The model under review builds one solid part; all positions refer to its coordinate system, in mm. Face numbers are marked on the shaded views. A direction names the side the tool comes from. Give positions to 0.01 mm unless a question says otherwise; leave off trailing zeros. Write each loop counter-clockwise with the first axis right and the second up, starting at its lowest first coordinate (ties: lowest second). Pieces come first, ordered by that corner, then holes. Notation, with made-up numbers: (80, 83) - (132, 83) arc R25 cw to (132, 101) - close; hole circle Ø11 at (33.25, 10.5). An arc over 180 degrees is marked (long way). Write item = value, one per line.
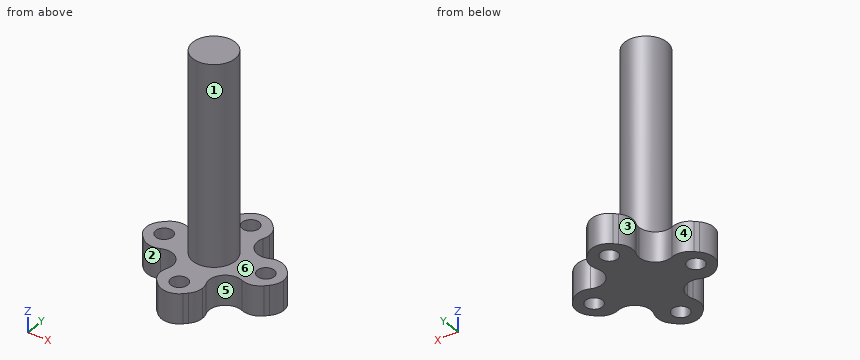
```python
from build123d import *

# Parameters (mm, degrees)
EXTRUDE_1_DEPTH = 3.5
SKETCH_3_R      = 2.5
EXTRUDE_2_DEPTH = 23.5


with BuildPart() as part:
    # 草图1 → 凸台-拉伸1 (new body)
    with BuildSketch(Plane.XY):
        with BuildLine():
            Line((-1.734039986, 7.089233915), (-1.356062107, 7.467211795))
            ThreePointArc((-1.356062107, 7.467211795), (0.128862134, 8.082287554), (1.613786374, 7.467211795))
            Line((1.613786374, 7.467211795), (1.991764254, 7.089233915))
            ThreePointArc((1.991764254, 7.089233915), (2.446987032, 6.407944883), (2.606840013, 5.604309675))
            ThreePointArc((2.606840013, 5.604309675), (2.564770676, 5.186073633), (2.440248217, 4.784594652))
            ThreePointArc((2.440248217, 4.784594652), (2.846019421, 2.699444842), (4.931169231, 2.293673637))
            ThreePointArc((4.931169231, 2.293673637), (6.152020505, 2.421597457), (7.235808495, 1.845189674))
            Line((7.235808495, 1.845189674), (7.613786374, 1.467211795))
            ThreePointArc((7.613786374, 1.467211795), (8.069009152, 0.785922762), (8.228862134, -0.017712446))
            ThreePointArc((8.228862134, -0.017712446), (8.069009152, -0.821347654), (7.613786374, -1.502636686))
            Line((7.613786374, -1.502636686), (7.235808495, -1.880614566))
            ThreePointArc((7.235808495, -1.880614566), (6.152020505, -2.457022348), (4.931169231, -2.329098529))
            ThreePointArc((4.931169231, -2.329098529), (2.846019421, -2.734869733), (2.440248217, -4.820019543))
            ThreePointArc((2.440248217, -4.820019543), (2.564770676, -5.221498525), (2.606840013, -5.639734566))
            ThreePointArc((2.606840013, -5.639734566), (2.446987032, -6.443369774), (1.991764254, -7.124658807))
            Line((1.991764254, -7.124658807), (1.613786374, -7.502636686))
            ThreePointArc((1.613786374, -7.502636686), (0.128862134, -8.117712446), (-1.356062107, -7.502636686))
            Line((-1.356062107, -7.502636686), (-1.734039986, -7.124658807))
            ThreePointArc((-1.734039986, -7.124658807), (-2.310447768, -6.040870817), (-2.182523949, -4.820019543))
            ThreePointArc((-2.182523949, -4.820019543), (-2.069860771, -4.456776655), (-2.031798038, -4.078372618))
            ThreePointArc((-2.031798038, -4.078372618), (-2.882781632, -2.494212089), (-4.673444964, -2.329098529))
            ThreePointArc((-4.673444964, -2.329098529), (-5.894296238, -2.457022348), (-6.978084227, -1.880614566))
            Line((-6.978084227, -1.880614566), (-7.356062107, -1.502636686))
            ThreePointArc((-7.356062107, -1.502636686), (-7.971137866, -0.017712446), (-7.356062107, 1.467211795))
            Line((-7.356062107, 1.467211795), (-6.978084227, 1.845189674))
            ThreePointArc((-6.978084227, 1.845189674), (-5.894296238, 2.421597457), (-4.673444964, 2.293673637))
            ThreePointArc((-4.673444964, 2.293673637), (-2.882781632, 2.458787198), (-2.031798038, 4.042947726))
            ThreePointArc((-2.031798038, 4.042947726), (-2.069860771, 4.421351764), (-2.182523949, 4.784594652))
            ThreePointArc((-2.182523949, 4.784594652), (-2.310447768, 6.005445926), (-1.734039986, 7.089233915))
        make_face()
        with BuildLine():
            ThreePointArc((-0.871137866, 5.982287554), (0.128862134, 4.982287554), (1.128862134, 5.982287554))
            ThreePointArc((1.128862134, 5.982287554), (0.128862134, 6.982287554), (-0.871137866, 5.982287554))
        make_face(mode=Mode.SUBTRACT)
        with BuildLine():
            ThreePointArc((-0.871137866, -6.017712446), (0.128862134, -7.017712446), (1.128862134, -6.017712446))
            ThreePointArc((1.128862134, -6.017712446), (0.128862134, -5.017712446), (-0.871137866, -6.017712446))
        make_face(mode=Mode.SUBTRACT)
        with BuildLine():
            ThreePointArc((5.128862134, -0.017712446), (6.128862134, -1.017712446), (7.128862134, -0.017712446))
            ThreePointArc((7.128862134, -0.017712446), (6.128862134, 0.982287554), (5.128862134, -0.017712446))
        make_face(mode=Mode.SUBTRACT)
        with BuildLine():
            ThreePointArc((-6.871137866, -0.017712446), (-5.871137866, -1.017712446), (-4.871137866, -0.017712446))
            ThreePointArc((-4.871137866, -0.017712446), (-5.871137866, 0.982287554), (-6.871137866, -0.017712446))
        make_face(mode=Mode.SUBTRACT)
    extrude(amount=EXTRUDE_1_DEPTH)

    # 草图3 → 凸台-拉伸2 (add)
    with BuildSketch(Plane.XY.offset(3.5)):
        Circle(SKETCH_3_R)
    extrude(amount=EXTRUDE_2_DEPTH)


solid = part.part
```
1. For line 1 (Z direction, x = 3.25, y = -2); line 2 (Y direction, x = 0.75, z = 3.25); line 3 (Y direction, x = -1.75, z = 21.75), list the stretches that pass through material, from the lowest coordinate up. Write a range as from..to.
Findings below:
line_1 = 0..3.5
line_2 = -8.02..-6.8, -5.23..5.2, 6.77..7.99
line_3 = -1.79..1.79
2. Take a section at D-D on z = 6.5. Give the boundary of the cut face in (x, y), and give its area (3 significant figures).
Findings below:
outline = circle Ø5 at (0, 0)
area = 19.6 mm²
3. Machinability: for the marked faces 1 and 2, which of the approach directions +Z, -Z, +X, -X, +Y, -Y give a long, thin tool a straight path to every point of the face, cutting with its end or side? Answer none if there is none.
Findings below:
face_1 = +Z
face_2 = +Z, -Z, -Y
4. Insertion check: P1, Ø3, axis at x = -5.87, y = -0.02, coming from the +Z side; P2, Ø6, axis at x = 0.5, z = 20, coming from the +Y side; P3, Ø1, axis at y = -1, z = 13.5, coming from the +X side. Each pin has a flat end and moves straight along its axis. Give the tip position at first contact, or say it passes through.
Findings below:
P1 = 3.5
P2 = 2.5
P3 = 2.45
5. Take a section at A-A on z = 3. Give the boundary of the cut face in (x, y).
Findings below:
outline = (-7.36, -1.5) - (-6.98, -1.88) arc R2.1 ccw to (-4.67, -2.33) arc R1.9 cw to (-2.18, -4.82) arc R2.1 ccw to (-1.73, -7.12) - (-1.36, -7.5) arc R2.1 ccw to (1.61, -7.5) - (1.99, -7.12) arc R2.1 ccw to (2.44, -4.82) arc R1.9 cw to (4.93, -2.33) arc R2.1 ccw to (7.24, -1.88) - (7.61, -1.5) arc R2.1 ccw to (7.61, 1.47) - (7.24, 1.85) arc R2.1 ccw to (4.93, 2.29) arc R1.9 cw to (2.44, 4.78) arc R2.1 ccw to (1.99, 7.09) - (1.61, 7.47) arc R2.1 ccw to (-1.36, 7.47) - (-1.73, 7.09) arc R2.1 ccw to (-2.18, 4.78) arc R1.9 cw to (-4.67, 2.29) arc R2.1 ccw to (-6.98, 1.85) - (-7.36, 1.47) arc R2.1 ccw to start; hole circle Ø2 at (-5.87, -0.02); hole circle Ø2 at (0.13, -6.02); hole circle Ø2 at (0.13, 5.98); hole circle Ø2 at (6.13, -0.02)
6. Take a section at B-B on x = 0.5. Give the boundary of the cut face in (y, z).
Findings below:
outline = (-8.08, 0) - (-6.95, 0) - (-6.95, 3.5) - (-8.08, 3.5) - close; (-5.09, 0) - (5.05, 0) - (5.05, 3.5) - (2.45, 3.5) - (2.45, 27) - (-2.45, 27) - (-2.45, 3.5) - (-5.09, 3.5) - close; (6.91, 0) - (8.05, 0) - (8.05, 3.5) - (6.91, 3.5) - close
7. Take a section at C-C on y = 3.5. Give the boundary of the cut face in (x, z).
Findings below:
outline = (-2.11, 0) - (2.37, 0) - (2.37, 3.5) - (-2.11, 3.5) - close
8. Draft analysis for pull direction Y (two halves, no side actions). For the marked faces 3, 4, 5 and 6, state which applies: +Y half, -Y half, draft (parallel to the pull), parting line (faces both ways), or undercut.
Findings below:
face_3 = undercut
face_4 = +Y half
face_5 = undercut
face_6 = draft
